Autodesk Inventor part; units mm, degrees
ref_plane "Plano de trabajo1" through (0, -526.2, 0) normal (1, 0, 0) x (0, 0, -1)
ref_plane "YZ Plane" through (0, 0, 0) normal (1, 0, 0) x (0, 1, 0)
ref_plane "XZ Plane" through (0, 0, 0) normal (0, 1, 0) x (-1, 0, 0)
sketch "Boceto1" plane through (0, 0, 0) normal (0, 0, 1) x (1, 0, 0)
  line L0 (300, -450) -> (-300, -450)
  line L1 (-300, -450) -> (-300, 450)
  line L2 (-300, 450) -> (300, 450)
  line L3 (300, 450) -> (300, -450)
  line L4 (300, -450) -> (-300, 450) construction
  line L5 (-300, -450) -> (300, 450) construction
  line L6 (376.2, 526.2) -> (-376.2, 526.2)
  line L7 (-376.2, 526.2) -> (-376.2, -526.2)
  line L8 (-376.2, -526.2) -> (376.2, -526.2)
  line L9 (376.2, -526.2) -> (376.2, 526.2)
  line L10 (-300, -450) -> (-300, -526.2)
  line L11 (300, -450) -> (300, -526.2)
  line L12 (300, 450) -> (300, 526.2)
  line L13 (-300, 450) -> (-300, 526.2)
  line L14 (-300, -450) -> (-376.2, -450)
  line L15 (300, -450) -> (376.2, -450)
  point P0 (0, 0)
  dimension "d0" = 600
  dimension "d1" = 900
  dimension "d2" = 76.2
extrude "Extrusión1" add sketch "Boceto1" along normal blind 76.2 contours L11 L8 L10 L0 | L15 L9 L8 L11 | L3 L12 L6 L9 L15 | L14 L7 L6 L13 L1 | L10 L8 L7 L14 | L2 L13 L6 L12
extrude "Extrusión2" add sketch "Boceto1" along normal blind 1200 contours L15 L9 L8 L11 | L10 L8 L7 L14
sketch "Boceto2" plane through (300, -450, 76.2) normal (0, 1, 0) x (1, 0, 0)
  line L0 (76.2, 0) -> (76.2, -1123.8)
  line L1 (76.2, -1123.8) -> (76.2, -973.8)
  line L2 (76.2, -973.8) -> (0, -973.8)
  line L3 (0, 0) -> (0, -1123.8)
  line L4 (76.2, -973.8) -> (76.2, -897.6)
  line L5 (76.2, -897.6) -> (0, -897.6)
  line L6 (0, -897.6) -> (0, -973.8)
  line L7 (-600, 0) -> (-600, -1123.8)
  line L8 (-600, -897.6) -> (-600, -973.8)
  line L9 (-676.2, 0) -> (-676.2, -1123.8)
  line L10 (-676.2, -973.8) -> (-676.2, -897.6)
  line L11 (-600, -897.6) -> (-676.2, -897.6)
  line L12 (-600, -973.8) -> (-676.2, -973.8)
  point P0 (-300, 76.2)
  dimension "d7" = 150
  dimension "d8" = 76.2
extrude "Extrusión3" add sketch "Boceto2" along normal blind 350
sketch "Boceto3" plane through (376.2, -526.2, 0) normal (1, 0, 0) x (0, 0, -1)
  line L0 (0, 0) -> (0, 1052.4)
  line L1 (0, 1052.4) -> (-76.2, 1052.4)
  line L2 (-76.2, 76.2) -> (-76.2, 1052.4)
  line L3 (-76.2, 76.2) -> (-973.8, 76.2)
  line L4 (-973.8, 76.2) -> (-973.8, 426.2)
  line L5 (-1050, 426.2) -> (-973.8, 426.2)
  line L6 (-1050, 76.2) -> (-1050, 426.2)
  line L7 (-1050, 76.2) -> (-1200, 76.2)
  line L8 (-1200, 0) -> (-1200, 76.2)
  line L9 (0, 0) -> (-1200, 0)
  circle A0 centre (-1011.9, 375.4) radius 25.4
  line L10 (-1011.9, 375.4) -> (-1011.9, 426.2)
  line L11 (-973.8, 426.2) -> (-1050, 426.2)
  circle A1 centre (-1011.9, 375.4) radius 25.4
  circle A2 centre (-1011.9, 375.4) radius 33.4
  point P0 (0, 526.2)
  dimension "d11" = 50.8
  dimension "d12" = 50.8
  dimension "d16" = 8
extrude "Extrusión4" cut sketch "Boceto3" against normal blind 1200 contours A0
shell "Vaciado1" thickness 2 removed faces 2 at (325.4, -152.8439, 986.5824) at (-350.8, -152.8439, 986.5824)
extrude "Extrusión5" add sketch "Boceto3" against normal blind 76.2 contours A2
sketch "Boceto4" plane through (-376.2, -526.2, 0) normal (-1, 0, 0) x (0, 0, 1)
  circle A0 centre (1011.9, 375.4) radius 33.4
  circle A1 centre (1011.9, 375.4) radius 25.4
  point P0 (0, 526.2)
extrude "Extrusión6" add sketch "Boceto4" against normal blind 76.2
extrude "Extrusión7" add sketch "Boceto3" along normal blind 8.8 contours A2
extrude "Extrusión8" add sketch "Boceto4" along normal blind 8.8
sketch "Boceto5" plane through (376.2, -450, 973.8) normal (0, 0, -1) x (-1, 0, 0)
  point P0 (376.2, 450)
sketch "Boceto6" plane through (0, 0, 1200) normal (0, 0, 1) x (1, 0, 0)
  line L0 (374.2, -452) -> (302, -452)
  line L1 (302, -452) -> (302, -524.2)
  line L2 (374.2, -524.2) -> (374.2, -452)
  line L3 (302, -524.2) -> (374.2, -524.2)
  line L4 (300, -526.2) -> (376.2, -526.2)
  line L5 (300, -450) -> (300, -526.2)
  line L6 (300, -526.2) -> (376.2, -526.2)
  line L7 (376.2, -526.2) -> (376.2, -450)
  line L8 (376.2, -450) -> (300, -450)
  line L9 (-376.2, -450) -> (-376.2, -526.2)
  line L10 (-376.2, -526.2) -> (-300, -526.2)
  line L11 (-300, -526.2) -> (-300, -450)
  line L12 (-300, -450) -> (-376.2, -450)
  line L13 (-302, -452) -> (-374.2, -452)
  line L14 (-302, -524.2) -> (-302, -452)
  line L15 (-374.2, -452) -> (-374.2, -524.2)
  line L16 (-374.2, -524.2) -> (-302, -524.2)
  point P0 (0, 0)
extrude "Extrusión9" cut sketch "Boceto6" against normal blind 2 contours L2 L3 L1 L0 | L14 L16 L15 L13
sketch "Boceto7" plane through (300, -100, 76.2) normal (0, 1, 0) x (1, 0, 0)
  line L0 (-600, -973.8) -> (-600, -897.6)
  line L1 (-600, -897.6) -> (-676.2, -897.6)
  line L2 (-676.2, -897.6) -> (-676.2, -973.8)
  line L3 (-676.2, -973.8) -> (-600, -973.8)
  line L4 (-674.2, -899.6) -> (-674.2, -971.8)
  line L5 (-674.2, -971.8) -> (-602, -971.8)
  line L6 (-602, -899.6) -> (-674.2, -899.6)
  line L7 (-602, -971.8) -> (-602, -899.6)
  line L8 (0, -897.6) -> (0, -973.8)
  line L9 (0, -973.8) -> (76.2, -973.8)
  line L10 (76.2, -973.8) -> (76.2, -897.6)
  line L11 (76.2, -897.6) -> (0, -897.6)
  line L12 (2, -899.6) -> (2, -971.8)
  line L13 (2, -971.8) -> (74.2, -971.8)
  line L14 (74.2, -899.6) -> (2, -899.6)
  line L15 (74.2, -971.8) -> (74.2, -899.6)
  point P0 (-300, 76.2)
extrude "Extrusión10" cut sketch "Boceto7" against normal blind 2 contours L6 L7 L5 L4 | L14 L15 L13 L12
sketch "Boceto8" plane through (-376.2, -450, 1200) normal (0, 1, 0) x (1, 0, 0)
  point P0 (376.2, 1200)
sketch "Boceto9" plane through (376.2, -526.2, 0) normal (1, 0, 0) x (0, 0, -1)
  line L0 (-1200, 74.2) -> (-1200, 2)
  line L1 (-1200, 38.1) -> (-1174.6, 38.1)
  point P0 (0, 526.2)
  dimension "d29" = 25.4
ref_plane "Plano de trabajo1" through (0, -526.2, 0) normal (1, 0, 0) x (0, 0, -1)
sketch "Boceto12" plane through (376.2, -526.2, 0) normal (1, 0, 0) x (0, 0, -1)
  line L0 (0, 0) -> (-1200, 0)
  line L1 (-1050, 76.2) -> (-1200, 76.2)
  line L2 (-1200, 0) -> (-1123.8, 0)
  line L3 (-1123.8, 0) -> (-1123.8, 76.2)
  line L4 (-1123.8, 76.2) -> (-1200, 76.2)
  line L5 (-1200, 76.2) -> (-1200, 0)
  circle A0 centre (-1192.6591, 7.3409) radius 4
  circle A1 centre (-1131.1409, 7.3409) radius 4
  circle A2 centre (-1131.1409, 68.8591) radius 4
  circle A3 centre (-1192.6591, 68.8591) radius 4
  point P0 (0, 526.2)
  dimension "d30" = 76.2
  dimension "d32" = 8
  dimension "d33" = 8
  dimension "d34" = 8
  dimension "d35" = 8
extrude "Extrusión11" cut sketch "Boceto12" against normal blind 770 contours A0 | A1 | A2 | A3
sketch "Boceto13" plane through (-300, -526.2, 76.2) normal (1, 0, 0) x (0, 0, -1)
  line L0 (-1123.8, 76.2) -> (-1123.8, 0)
  line L1 (-973.8, 76.2) -> (-1123.8, 76.2)
  line L2 (-1123.8, 0) -> (-1047.6, 0)
  line L3 (-1047.6, 0) -> (-1047.6, 76.2)
  line L4 (-1047.6, 76.2) -> (-1123.8, 76.2)
  line L5 (-1123.8, 76.2) -> (-1123.8, 0)
  line L6 (-973.8, 76.2) -> (-1123.8, 76.2)
  line L7 (-1047.6, 0) -> (-1007.6, 0)
  line L8 (-1007.6, 0) -> (-1007.6, 76.2)
  line L9 (-1007.6, 76.2) -> (-1047.6, 76.2)
  line L10 (-1047.6, 76.2) -> (-1047.6, 0)
  point P0 (76.2, 526.2)
  point P1 (-1007.6, 76.2)
  dimension "d38" = 76.2
  dimension "d39" = 40
extrude "Extrusión12" add sketch "Boceto13" along normal blind 8 contours L1 L8 L7 L3
sketch "Boceto14" plane through (300, -526.2, 76.2) normal (-1, 0, 0) x (0, 0, 1)
  line L0 (1007.6, 76.2) -> (1007.6, 0)
  line L1 (1047.6, 0) -> (1047.6, 76.2)
  circle A0 centre (1054.9409, 68.8591) radius 4
  circle A1 centre (1054.9409, 7.3409) radius 4
  circle A2 centre (1116.4591, 68.8591) radius 4
  circle A3 centre (1116.4591, 7.3409) radius 4
  circle A4 centre (935.7, 375.4) radius 25.4
  line L2 (0, 0) -> (0, 76.2)
  line L3 (0, 0) -> (1123.8, 0)
  line L4 (1123.8, 76.2) -> (1123.8, 0)
  line L5 (973.8, 76.2) -> (1123.8, 76.2)
  line L6 (973.8, 76.2) -> (973.8, 426.2)
  line L7 (897.6, 426.2) -> (973.8, 426.2)
  line L8 (897.6, 76.2) -> (897.6, 426.2)
  line L9 (0, 76.2) -> (897.6, 76.2)
  point P0 (-76.2, 526.2)
extrude "Extrusión13" add sketch "Boceto14" along normal blind 8 contours L5 L1 L3 L0
properties part number "Principal"
Model file for the job. Use its own axes, mm. A direction names the side the tool comes from. Round coordinates to 2 decimals unless told otherwise and drop trailing zeros. Order: outer loops, then holes, each group sorted by start corner. A loop starts at its lowest first (then second) coordinate and runs counter-clockwise, first axis right, second up.
(1) 3-axis set-ups, long thin cutter, end or side, ignore diameter. For faces 1 (the face through (-341.1, -100, 1048.4)), 2 (the face through (-338.61, -171.12, 985.39)), 3 (the face through (300, -488, 1161)), 4 (the face through (338, -450, 519)): which of +Z, -Z, +X, -X, +Y, -Y reach the whole face in a straight line?
(2) Drill centre lines: line 1 (X direction, y = -469.5, z = 526); line 2 (Y direction, x = 318, z = 1011.9); line 3 (Y direction, x = 318, z = 1085). Where is each one in solid material? Low to high.
(3) Band-saw the part on A-A (y = 292). List the corners of the cut face in (x, z), then the cut area to 3 significant figures.
(4) Band-saw the part on B-B (x = 216). List the corners of the cut face in (y, z), then the cut area to 3 significant figures.
(5) Pin check, flat tips, straight feed: pin 1 (2 mm diameter, centred on y = -118, z = 1020.5, fed in from +X); pin 2 (4 mm diameter, centred on x = 294, z = 1095, fed in from +Y); pin 3 (9 mm diameter, centred on x = 294.5, y = -488, fed in from +Z). Stop position of each tip, or through.
(6) Band-saw the part on C-C (y = -434.5). Give the number of separate pieces and of enclosed holes in the cut face, then the cut area to 3 significant figures.
(7) Pull direction Y, two halves, no side cores. Call faces 5 (the face through (-338, -277, 1050)), 6 (the face through (338, -452, 519)), 7 (the face through (4, -450, 38)), 8 (the face through (-380.538, -152.269, 978.532)): released by +Y, released by -Y, zero draft, split by the parting line, or undercut.
Verdict:
1. face 1: +Z, +X, -X, +Y
1. face 2: none
1. face 3: +Z, +Y, -Y
1. face 4: +X, -X, +Y
2. line 1: x = -376.2 to -374.2, -302 to -300, 300 to 302, 374.2 to 376.2
2. line 2: y = -526.2 to -524.2, -184.2 to -176.2, -125.4 to -117.4
2. line 3: y = -526.2 to -524.2, -452 to -450
3. outline: (-376.2, 0) - (-300, 0) - (-300, 76.2) - (-376.2, 76.2) - close; (300, 0) - (376.2, 0) - (376.2, 76.2) - (300, 76.2) - close; hole (-374.2, 2) - (-302, 2) - (-302, 74.2) - (-374.2, 74.2) - close; hole (302, 2) - (374.2, 2) - (374.2, 74.2) - (302, 74.2) - close
3. area: 1,190 mm2
4. outline: (-526.2, 0) - (-450, 0) - (-450, 76.2) - (-526.2, 76.2) - close; (450, 0) - (526.2, 0) - (526.2, 76.2) - (450, 76.2) - close; hole (-524.2, 2) - (-452, 2) - (-452, 74.2) - (-524.2, 74.2) - close; hole (452, 2) - (524.2, 2) - (524.2, 74.2) - (452, 74.2) - close
4. area: 1,190 mm2
5. pin 1: stops at x = 385
5. pin 2: stops at y = -450
5. pin 3: stops at z = 1123.8
6. separate pieces: 4
6. enclosed holes: 4
6. area: 2,370 mm2
7. face 5: zero draft
7. face 6: undercut
7. face 7: undercut
7. face 8: split by the parting line
